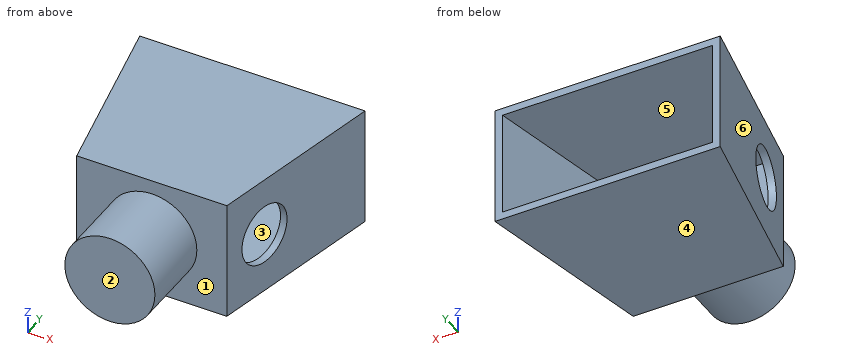
from build123d import *

# Parameters (mm, degrees)
F1_DEPTH = 8
F2_T     = -0.5
F3_R     = 3
F4_DEPTH = 5
F5_R     = 2
F6_DEPTH = 5


# Not quite as in the source:
# - a pattern or mirror of a feature is missing from the dataset's text; its kind, count and spacing are read off the source's solid


with BuildPart() as f1:
    # F0 (on Top) → F1 (new body)
    with BuildSketch(Plane.XY):
        Polygon((-7.5, 0), (-5, -12), (5, -12), (7.5, 0), align=None)
    extrude(amount=F1_DEPTH)

    # F2
    f2_openings = [f1.faces().sort_by_distance(p)[0] for p in [
        (0, 0, 4),
    ]]
    offset(amount=F2_T, openings=f2_openings)

    # F3 (on face) → F4 (join)
    with BuildSketch(Plane.XZ.offset(12)):
        with Locations((0, 4.0601608343)):
            Circle(F3_R)
    extrude(amount=F4_DEPTH)

    # F5 (on face) → F6 (cut)
    with BuildSketch(Plane(origin=(7.1880199667, -1.4975041597, 0), x_dir=(0.2039542541, 0.9789804197, 0), z_dir=(0.9789804197, -0.2039542541, 0))):
        with Locations((-7.3930048384, 4.0684221312)):
            Circle(F5_R)
    f6 = extrude(amount=-F6_DEPTH, mode=Mode.SUBTRACT)

    # F6_copies: F6 across plane
    add(f6.mirror(Plane(origin=(0, 0, 0), x_dir=(0, 0, -1), z_dir=(-1, 0, 0))), mode=Mode.SUBTRACT)


solid = f1.part
Check sheet for the modelled part. Datum: model origin and axes. Units: mm. Face numbers are marked on the shaded views. A direction names the side the tool comes from. Give positions to 0.01 mm unless a question says otherwise; leave off trailing zeros. Write each loop counter-clockwise with the first axis right and the second up, starting at its lowest first coordinate (ties: lowest second). Pieces come first, ordered by that corner, then holes. Notation, with made-up numbers: (24, -19) -> (81, -19) arc R28 cw to (81, 11) -> close; hole circle Ø1 at (23, 20). An arc over 180 degrees is marked (long way). One line per item, written item: value. Start each with the question number.
Item 1: Draft check along Z on the marked faces 4, 5 and 6. Enter one of: +Z half, -Z half, draft (parallel to the pull), parting line (faces both ways), or undercut.
Item 2: Section check B-B on x = 0. Record the cut outline in (y, z), then the cut area to 3 significant figures.
Item 3: Material ranges on probe 1 along Z at (x, y) = (-3.25, -8.75); probe 2 along Y at (x, z) = (-4.5, 4.5); probe 3 along Y at (x, z) = (-4.75, 7.75), recorded low to high. Write a range as from..to.
Item 4: Section check C-C on y = -11.25. Record the cut outline in (x, z).
Item 5: Section check D-D on z = 2.5. Record the cut outline in (x, y), then the cut area to 3 significant figures.
Item 6: Tool access check on the marked faces 1, 2 and 3. Record the directions out of +Z, -Z, +X, -X, +Y, -Y that give a thin tool (end or side, any length) a straight path to the whole face; none if there is none.
Item 7: Gauge pin test, flat ends, axial feed: pin 1 (3.5 mm diameter, centred on x = -0.5, z = 3.5, fed in from +Y); pin 2 (2 mm diameter, centred on y = -7.5, z = 5.5, fed in from +X). Record the tip position at first contact, or that the pin passes through.
Item 8: Section check A-A on z = 3.75. Record the cut outline in (x, y).
Results list:
1. face 4: -Z half
1. face 5: undercut
1. face 6: draft
2. outline: (-17, 1.06) -> (-12, 1.06) -> (-12, 0) -> (0, 0) -> (0, 0.5) -> (-11.5, 0.5) -> (-11.5, 7.5) -> (0, 7.5) -> (0, 8) -> (-12, 8) -> (-12, 7.06) -> (-17, 7.06) -> close
2. area: 45.5 mm²
3. probe 1: 0..0.5, 7.5..8
3. probe 2: -12..-11.5
3. probe 3: -12..0
4. outline: (-5.16, 0) -> (5.16, 0) -> (5.16, 8) -> (-5.16, 8) -> close; hole (-4.65, 0.5) -> (4.65, 0.5) -> (4.65, 7.5) -> (-4.65, 7.5) -> close
5. outline: (-7.5, 0) -> (-5.93, -7.52) -> (-5.44, -7.42) -> (-6.99, 0) -> close; (-5.43, -9.95) -> (-5, -12) -> (-2.56, -12) -> (-2.56, -17) -> (2.56, -17) -> (2.56, -12) -> (5, -12) -> (5.43, -9.95) -> (4.94, -9.85) -> (4.59, -11.5) -> (-4.59, -11.5) -> (-4.94, -9.85) -> close; (5.44, -7.42) -> (5.93, -7.52) -> (7.5, 0) -> (6.99, 0) -> close
5. area: 39.9 mm²
6. face 1: -Y
6. face 2: +Z, -Z, +X, -X, -Y
6. face 3: +Y
7. pin 1: y = -11.5
7. pin 2: x = 6.15
8. outline: (-7.5, 0) -> (-6.08, -6.8) -> (-5.59, -6.7) -> (-6.99, 0) -> close; (-5.28, -10.67) -> (-5, -12) -> (-2.98, -12) -> (-2.98, -17) -> (2.98, -17) -> (2.98, -12) -> (5, -12) -> (5.28, -10.67) -> (4.79, -10.57) -> (4.59, -11.5) -> (-4.59, -11.5) -> (-4.79, -10.57) -> close; (5.59, -6.7) -> (6.08, -6.8) -> (7.5, 0) -> (6.99, 0) -> close
